Could you check a few things on this drawing? It's one solid part, dimensions in mm from its lowest x, y, z. Give positions to 0.01 mm unless a question says otherwise; leave off trailing zeros. Order: outer loops, then holes, each group sorted by start corner. A loop starts at its lowest first (then second) coordinate and runs counter-clockwise, first axis right, second up. Notation, with made-up numbers: (27, 8) - (62, 8) arc R8 cw to (62, 22) - close; hole circle Ø2 at (-39.5, 10.5). An arc over 180 degrees is marked (long way). Return JSON: item names as keys, results as strings.
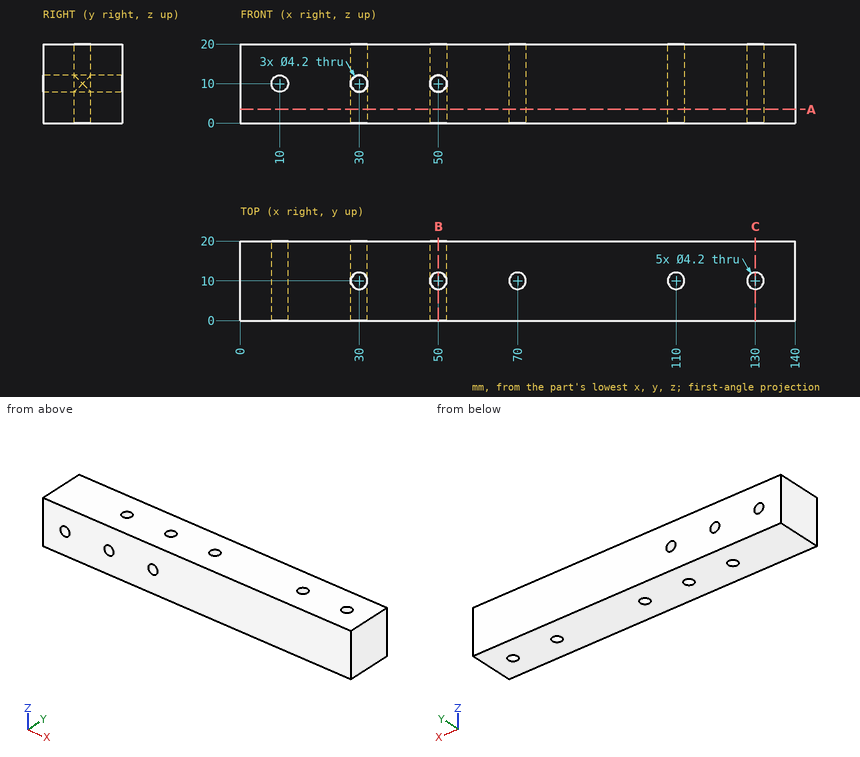
1. Suppose I cut it at A-A (z = 3.5). List the corners of the cut face in (x, y) for me.
Checks:
{"outline": "(0, 0) - (140, 0) - (140, 20) - (0, 20) - close; hole circle Ø4.2 at (30, 10); hole circle Ø4.2 at (50, 10); hole circle Ø4.2 at (70, 10); hole circle Ø4.2 at (110, 10); hole circle Ø4.2 at (130, 10)"}
2. For pin 1 Ø2 at (y, z) = (5.5, 6.5) entering from -X, with a flat end and sliding along its axis, tell me the tip position at first contact or that it passes through.
Checks:
{"pin 1": "x = 0"}
3. If I drill on L1, parallel to X at y = 2, z = 9.75; L2, parallel to Y at x = 50, z = 3.25; L3, parallel to X at y = 10.75, z = 4, over which ranges is the centre line in solid material (lowest first)? Write a range as [from, to].
Checks:
{"L1": "[0, 7.91], [12.09, 27.91], [32.09, 47.91], [52.09, 140]", "L2": "[0, 7.9], [12.1, 20]", "L3": "[0, 28.04], [31.96, 48.04], [51.96, 68.04], [71.96, 108.04], [111.96, 128.04], [131.96, 140]"}
4. Suppose I cut it at C-C (x = 130). List the corners of the cut face in (y, z) for me.
Checks:
{"outline": "(0, 0) - (7.9, 0) - (7.9, 20) - (0, 20) - close; (12.1, 0) - (20, 0) - (20, 20) - (12.1, 20) - close"}
5. Suppose I cut it at B-B (x = 50). List the corners of the cut face in (y, z) for me, plus the area to 3 significant figures.
Checks:
{"outline": "(0, 0) - (7.9, 0) - (7.9, 7.9) - (0, 7.9) - close; (0, 12.1) - (7.9, 12.1) - (7.9, 20) - (0, 20) - close; (12.1, 0) - (20, 0) - (20, 7.9) - (12.1, 7.9) - close; (12.1, 12.1) - (20, 12.1) - (20, 20) - (12.1, 20) - close", "area": "250 mm^2"}
